from build123d import *

# Parameters (mm, degrees)
CUT_EXTRUDE_START   = -3.5
CUT_EXTRUDE_1_DEPTH = 10
SKETCH_3_W          = 4
SKETCH_3_H          = 19.670556204
CUT_EXTRUDE_2_DEPTH = 10
CUT_EXTRUDE_START_2 = -29
SKETCH_4_R          = 4
SKETCH_4_R_2        = 2
CUT_EXTRUDE_3_DEPTH = 29
SKETCH_5_R          = 1
CUT_EXTRUDE_4_DEPTH = 5
SKETCH_6_R          = 2
EXTRUDE_1_DEPTH     = 1
EXTRUDE_START       = -4.5
SKETCH_7_R          = 2.5
SKETCH_7_R_2        = 2
EXTRUDE_2_DEPTH     = 1
CHAMFER_2_SIZE      = 0.25
SKETCH_8_R          = 2
EXTRUDE_3_DEPTH     = 0.5
SKETCH_11_R         = 1.5
EXTRUDE_4_DEPTH     = 5


with BuildPart() as part:
    # 草图1 → 旋转2 (revolve)
    with BuildSketch(Plane.XY, mode=Mode.PRIVATE) as revolve_2_sk:
        Polygon((0, 2), (0, 0), (17, 0), (21, 0), (21, 2), (17, 2), (17, 4), (4, 4), (4, 2), align=None)
    revolve(revolve_2_sk.sketch.rotate(Axis((-16.701754386, 0, 0), (1, 0, 0)), 180), axis=Axis((-16.701754386, 0, 0), (1, 0, 0)))

    # 草图2 → 切除-拉伸1 (cut)
    with BuildSketch(Plane.XY.offset(CUT_EXTRUDE_START)):
        Polygon((12.5, -5.827233832), (12.5, 4), (10.5, 4), (8.5, 4), (8.5, -5.827233832), align=None)
    extrude(amount=-CUT_EXTRUDE_1_DEPTH, mode=Mode.SUBTRACT)

    # 草图3 → 切除-拉伸2 (cut)
    with BuildSketch(Plane(origin=(0, 0, 0), x_dir=(1, 0, 0), z_dir=(0, 1, 0)).offset(CUT_EXTRUDE_START)):
        with Locations((10.5, 3.5)):
            Rectangle(SKETCH_3_W, SKETCH_3_H)
    extrude(amount=-CUT_EXTRUDE_2_DEPTH, mode=Mode.SUBTRACT)

    # 草图4 → 切除-拉伸3 (cut)
    with BuildSketch(Plane(origin=(21, 0, 0), x_dir=(0, 0, -1), z_dir=(1, 0, 0)).offset(CUT_EXTRUDE_START_2)):
        Circle(SKETCH_4_R)
        with Locations(Location((0, 0, 0), (0, 0, 270))):
            Circle(SKETCH_4_R_2, mode=Mode.SUBTRACT)
    extrude(amount=CUT_EXTRUDE_3_DEPTH, mode=Mode.SUBTRACT)

    # 草图5 → 切除-拉伸4 (cut, symmetric)
    with BuildSketch(Plane.XY):
        with Locations((10.5, 0)):
            Circle(SKETCH_5_R)
    extrude(amount=CUT_EXTRUDE_4_DEPTH, both=True, mode=Mode.SUBTRACT)

    # 草图6 → 凸台-拉伸1 (add)
    with BuildSketch(Plane(origin=(21, 0, 0), x_dir=(0, 0, -1), z_dir=(1, 0, 0))):
        with Locations(Location((0, 0, 0), (0, 0, 270))):
            Circle(SKETCH_6_R)
    extrude(amount=EXTRUDE_1_DEPTH)

    # 草图7 → 凸台-拉伸2 (add)
    with BuildSketch(Plane(origin=(22, 0, 0), x_dir=(0, 0, -1), z_dir=(1, 0, 0)).offset(EXTRUDE_START)):
        with Locations(Location((0, 0, 0), (0, 0, 90))):
            Circle(SKETCH_7_R)
        with Locations(Location((0, 0, 0), (0, 0, 270))):
            Circle(SKETCH_7_R_2, mode=Mode.SUBTRACT)
    extrude(amount=EXTRUDE_2_DEPTH)

    # 倒角2
    chamfer_2_edges = [part.edges().sort_by_distance(p)[0] for p in [
        (0, 2, 0),
    ]]
    chamfer(chamfer_2_edges, length=CHAMFER_2_SIZE)

    # 草图8 → 凸台-拉伸3 (add)
    with BuildSketch(Plane(origin=(22, 0, 0), x_dir=(0, 0, -1), z_dir=(1, 0, 0))):
        with Locations(Location((0, 0, 0), (0, 0, 270))):
            Circle(SKETCH_8_R)
    extrude(amount=EXTRUDE_3_DEPTH)

    # 草图11 → 凸台-拉伸4 (add)
    with BuildSketch(Plane(origin=(22.5, 0, 0), x_dir=(0, 0, -1), z_dir=(1, 0, 0))):
        with Locations(Location((0, 0, 0), (0, 0, 90))):
            Circle(SKETCH_11_R)
    extrude(amount=EXTRUDE_4_DEPTH)


solid = part.part
Verification items for the finished model (mm, model axes). A direction names the side the tool comes from. Round coordinates to 2 decimals unless told otherwise and drop trailing zeros. Order: outer loops, then holes, each group sorted by start corner. A loop starts at its lowest first (then second) coordinate and runs counter-clockwise, first axis right, second up. Notation, with made-up numbers: (56, -30.5) -> (83, -30.5) arc R23 cw to (83, 6.5) -> close; hole circle Ø9 at (-27.75, 23). An arc over 180 degrees is marked (long way). Put each result on its own line as item: value.
1) Material ranges on line 1 (X direction, y = 0, z = -0.5); line 2 (Y direction, x = 3.5, z = 0.1); line 3 (X direction, y = 1.5, z = -1.95), recorded low to high.
Final values:
line 1: x = 0 to 9.5, 11.5 to 27.5
line 2: y = -2 to 2
line 3: x = 17.5 to 18.5
2) Section check D-D (x = 11). Record the cut outline in (y, z), then the cut area to 3 significant figures.
Final values:
outline: (-0.87, -1.8) -> (-0.87, 1.8) arc R2 ccw to start; (0.87, -1.8) arc R2 ccw to (0.87, 1.8) -> close
area: 5.86 mm^2
3) Section check C-C (x = 16.25). Record the cut outline in (y, z).
Final values:
outline: circle Ø4 at (0, 0)
4) Section check B-B (z = 0). Record the cut outline in (x, y), then the cut area to 3 significant figures.
Final values:
outline: (0, -1.75) -> (0.25, -2) -> (17.5, -2) -> (17.5, -2.5) -> (18.5, -2.5) -> (18.5, -2) -> (22.5, -2) -> (22.5, -1.5) -> (27.5, -1.5) -> (27.5, 1.5) -> (22.5, 1.5) -> (22.5, 2) -> (18.5, 2) -> (18.5, 2.5) -> (17.5, 2.5) -> (17.5, 2) -> (0.25, 2) -> (0, 1.75) -> close; hole circle Ø2 at (10.5, 0)
area: 103 mm^2
5) Depth check by flat-ended pin: pin 1 (1.2 mm diameter, centred on x = 10.5, y = 0, fed in from +Z). Enter the tip coordinate at first touch or a pass-through.
Final values:
pin 1: passes through
6) Section check A-A (y = 0). Record the cut outline in (x, z).
Final values:
outline: (0, -1.75) -> (0.25, -2) -> (9.5, -2) -> (9.5, 2) -> (0.25, 2) -> (0, 1.75) -> close; (11.5, -2) -> (17.5, -2) -> (17.5, -2.5) -> (18.5, -2.5) -> (18.5, -2) -> (22.5, -2) -> (22.5, -1.5) -> (27.5, -1.5) -> (27.5, 1.5) -> (22.5, 1.5) -> (22.5, 2) -> (18.5, 2) -> (18.5, 2.5) -> (17.5, 2.5) -> (17.5, 2) -> (11.5, 2) -> close
7) Set-up check for faces 1 (the flat face through (17.5, -1, 2)), 2 (the flat face through (27.5, 0, 0)), 3 (the cylindrical face through (24.96, 1.43, 0.45)): record each of +Z, -Z, +X, -X, +Y, -Y from which the full face is reachable in a straight line by a thin tool's end or side.
Final values:
face 1: -X
face 2: +Z, -Z, +X, +Y, -Y
face 3: +X
8) Mould release check, pull along Y, two halves, no side actions. Record for faces 4 (the flat face through (18.5, -1, 2)), 5 (the cylindrical face through (11.04, 0.84, 0.03)), 6 (the cylindrical face through (20, 0, 2)): +Y half, -Y half, draft (parallel to the pull), parting line (faces both ways), or undercut.
Final values:
face 4: draft
face 5: undercut
face 6: parting line
